Could you check a few things on this model? Use its own coordinates, in mm. A direction names the side the tool comes from. Give positions to 0.01 mm unless a question says otherwise; leave off trailing zeros. Loops run counter-clockwise (first coordinate to the right, second up) from the corner with the lowest first, then second, coordinate; pieces in that order, holes last. Notation, with made-up numbers: M 9.25,86 L 34.25,86 A5 cw 34.25,94 Z; hole C -26,-3 d8. An arc over 180 degrees is marked long. Use a Markdown table: item, result. Add a question column.
1) We'd pull the mould along Y, two halves only. Please class faces 3 (the flat face through (31, -17.3, 10)), 4 (the cylindrical face through (32.26, -15.56, 4.08)): +Y half, -Y half, draft (parallel to the pull), parting line (faces both ways), or undercut.
2) Suppose I cut it at A-A on z = 3.75. Count the separate pieces of the cut face and the enclosed holes in it, and give its area (3 significant figures).
3) Suppose I cut it at B-B on x = -7. List the corners of the cut face in (y, z) for me.
4) If I drill on line 1 along Y through (x, z) = (31.04, 2.5); line 2 along Y through (x, z) = (-46.36, 5); line 3 along Z through (x, y) = (-39, 5), over which ranges is the centre line in solid material (lowest first)? Write a range as [from, to].
5) Which directions (+Z, -Z, +X, -X, +Y, -Y) give clear straight access to the entire face, cutting with the end or side of a thin tool? Please do faces 1 (the flat face through (-14, 1, 0)), 2 (the flat face through (31, 10.7, 10)).
6) Suppose I cut it at C-C on y = 19.5. List the corners of the cut face in (x, z) for me.
7) Will this pin go through, and if not, where does the flat tip stop? pin 1 Ø3 at (x, z) = (-30, 1) entering from +Y.
Solid Edge part; units mm, degrees
sketch "Sketch1" plane through (0, 0, 0) normal (0, 0, 1) x (1, 0, 0)
  line L0 (48.2908, -44) -> (-78.36, -44)
  line L1 (-78.36, -44) -> (-78.36, 44)
  line L2 (-78.36, 44) -> (48.2908, 44)
  line L3 (48.2908, 44) -> (48.2908, -44)
extrude "Protrusion1" add sketch "Sketch1" against normal blind 2
sketch "Sketch2" plane through (0, 0, 0) normal (0, 0, 1) x (1, 0, 0)
  circle A0 centre (-72.36, 38) radius 3
  circle A1 centre (-46.36, 38) radius 3
  circle A2 centre (-46.36, -28) radius 3
  circle A3 centre (-19.76, -20.8) radius 3.6
  circle A4 centre (-19.76, 27.46) radius 3.6
  circle A5 centre (31.04, -15.72) radius 3.6
  circle A6 centre (31.04, 12.22) radius 3.6
  circle A7 centre (-72.36, -28) radius 3
extrude "ExtrudedProtrusion_3" add sketch "Sketch2" along normal blind 10
hole "Hole_1" at (-46.36, -28, 10) direction (0, 0, -1) diameter 1.567 end up to next
hole "Hole1" at (-72.36, -28, 10) direction (0, 0, -1) diameter 1.567 end up to next
hole "Hole2" at (-72.36, 38, 10) direction (0, 0, -1) diameter 1.567 end up to next
hole "Hole3" at (-46.36, 38, 10) direction (0, 0, -1) diameter 1.567 end up to next
hole "Hole_5" at (31.04, 12.22, 10) direction (0, 0, -1) diameter 2.459 end up to next
hole "Hole4" at (31.04, -15.72, 10) direction (0, 0, -1) diameter 2.459 end up to next
hole "Hole5" at (-19.76, -20.8, 10) direction (0, 0, -1) diameter 2.459 end up to next
hole "Hole6" at (-19.76, 27.46, 10) direction (0, 0, -1) diameter 2.459 end up to next
Answer block:
| question | item | result |
|---|---|---|
| 1 | face 3 | draft |
| 1 | face 4 | undercut |
| 2 | separate pieces | 8 |
| 2 | enclosed holes | 8 |
| 2 | area | 249 mm^2 |
| 3 | outline | M -44,-2 L 44,-2 L 44,0 L -44,0 Z |
| 4 | line 1 | y = [-19.32, -16.95], [-14.49, -12.12], [8.62, 10.99], [13.45, 15.82] |
| 4 | line 2 | y = [-31, -28.78], [-27.22, -25], [35, 37.22], [38.78, 41] |
| 4 | line 3 | z = [-2, 0] |
| 5 | face 1 | +Z |
| 5 | face 2 | +Z, +X, -X, +Y, -Y |
| 6 | outline | M -78.36,-2 L 48.29,-2 L 48.29,0 L -78.36,0 Z |
| 7 | pin 1 | stops at y = 44 |
